from build123d import *

# Parameters (mm, degrees)
BOSS_EXTRUDE1_DEPTH = 20
FILLET1_R           = 50


with BuildPart() as part:
    # Sketch1 → Boss-Extrude1 (new body)
    with BuildSketch(Plane.XY):
        with BuildLine():
            Line((-482.666666667, 166), (-182.666666667, 166))
            Line((-182.666666667, 166), (-182.666666667, -84))
            ThreePointArc((-182.666666667, -84), (-124.088022904, -225.421356237), (17.333333333, -284))
            Line((17.333333333, -284), (167.333333333, -284))
            Line((167.333333333, -284), (167.333333333, -484))
            Line((167.333333333, -484), (-482.666666667, -484))
            Line((-482.666666667, -484), (-482.666666667, 166))
        make_face()
    extrude(amount=BOSS_EXTRUDE1_DEPTH)

    # Fillet1
    fillet1_edges = [part.edges().sort_by_distance(p)[0] for p in [
        (167.333333333, -284, 10),
    ]]
    fillet(fillet1_edges, radius=FILLET1_R)


solid = part.part
Input: part model. Units: mm. Frame: model coordinates. A direction names the side the tool comes from. Coordinates: 2 decimals unless noted, no trailing zeros. Loops run counter-clockwise (first coordinate to the right, second up) from the corner with the lowest first, then second, coordinate; pieces in that order, holes last. Notation, with made-up numbers: (40.5, -21.5) -> (52.5, -21.5) arc R12 cw to (52.5, 1.5) -> close; hole circle Ø2 at (18, 65). An arc over 180 degrees is marked (long way). One line per item, written item: value.
(1) Cut plane C-C (x = 54). Output: boundary loops of the cut face in (y, z), then the cut area to 3 significant figures.
Answer below:
outline: (-484, 0) -> (-284, 0) -> (-284, 20) -> (-484, 20) -> close
area: 4,000 mm2
(2) Ray query, line 1 along Y through (x, z) = (38, 12.75); line 2 along X through (y, z) = (-50, 3); line 3 along X through (y, z) = (-94.5, 7.75). Return the intervals inside material, ascending.
Answer below:
line 1: y = -484 to -284
line 2: x = -482.67 to -182.67
line 3: x = -482.67 to -182.39
(3) Cut plane A-A (z = 9.75). Output: boundary loops of the cut face in (x, y), then the cut area to 3 significant figures.
Answer below:
outline: (-482.67, -484) -> (167.33, -484) -> (167.33, -334) arc R50 ccw to (117.33, -284) -> (17.33, -284) arc R200 cw to (-182.67, -84) -> (-182.67, 166) -> (-482.67, 166) -> close
area: 273,000 mm2
(4) Set-up query: faces 1 (the face through (-225, -227, 0)), 2 (the face through (67, -284, 10)). Return all of +Z, -Z, +X, -X, +Y, -Y with unobstructed straight access to the full face (end or side cutting, diameter ignored); none if empty.
Answer below:
face 1: -Z, +X, -X, +Y, -Y
face 2: +Z, -Z, +X, +Y
(5) Pin query (flat end, axial travel): pin 1 Ø3 at (y, z) = (-59.5, 7.5) entering from +X. Return the tip coordinate at first contact, or that it passes through.
Answer below:
pin 1: stops at x = -182.67
(6) Cut plane B-B (y = 74.5). Output: boundary loops of the cut face in (x, z).
Answer below:
outline: (-482.67, 0) -> (-182.67, 0) -> (-182.67, 20) -> (-482.67, 20) -> close
